Verification items for the finished model (mm, model axes). A direction names the side the tool comes from. Coordinates: 2 decimals unless noted, no trailing zeros. Order: outer loops, then holes, each group sorted by start corner. A loop starts at its lowest first (then second) coordinate and runs counter-clockwise, first axis right, second up. Notation, with made-up numbers: (53, 62) -> (69, 62) arc R18 ccw to (69, 92) -> close; hole circle Ø11 at (87, 42). An arc over 180 degrees is marked (long way). Write each question's results on one line, items separated by ' | '. Start each with the question number.
(1) Thickness scan on probe 1 along Y at (x, z) = (0, -8); probe 2 along Z at (x, y) = (2.5, -19.5); probe 3 along Y at (x, z) = (-33, -1.25). Record the ranges inside material, lowest first. Write a range as [from, to].
(2) Set-up check for faces 1 (the flat face through (0, 0, -14)), 2 (the cylindrical face through (0, 1, -9)), 3 (the flat face through (16, -25, -2)): record each of +Z, -Z, +X, -X, +Y, -Y from which the full face is reachable in a straight line by a thin tool's end or side.
(3) Cross-section at C-C on z = -1.5. Enter the section's corners in (x, y) (3 decimals).
(4) Cross-section at A-A on y = 0. Enter the section's corners in (x, z).
(5) Cross-section at D-D on z = -9. Enter the section's corners in (x, y), and give its area (3 significant figures).
(6) Go/stop test with flat-tipped pins: pin 1 (2 mm diameter, centred on y = -24, z = -1.5, fed in from +X); pin 2 (5 mm diameter, centred on y = -19, z = -1.5, fed in from -X); pin 3 (1 mm diameter, centred on x = 8.5, y = 10, fed in from -Z); pin 4 (1.8 mm diameter, centred on x = -30.094, y = 17.375, fed in from -Z). Record where each tip stops, or that it passes through.
(7) Draft check along X on faces 4 (the flat face through (-1, 1, 0)), 5 (the cylindrical face through (-31.593, -17.309, -1.972)), 6 (the cylindrical face through (-9, -40, -2)), 7 (the cylindrical face through (28.595, 17.441, -1.972)). Enter one of: +X half, -X half, draft (parallel to the pull), parting line (faces both ways), or undercut.
Autodesk Inventor part; units mm, degrees
ref_plane "Work Plane3" through (0, 0, 0) normal (0, 0, 1) x (1, 0, 0)
ref_plane "Work Plane6" through (0, 0, -4) normal (0, 0, -1) x (-1, 0, 0)
ref_plane "YZ Plane" through (0, 0, 0) normal (1, 0, 0) x (0, 1, 0)
sketch "Sketch1" plane through (0, 0, 0) normal (0, 0, 1) x (1, 0, 0)
  circle A0 centre (0, 0) radius 41
  circle A1 centre (0, 0) radius 17.705
  circle A2 centre (0, 0) radius 15
  circle A3 centre (0, 15) radius 0.75
  circle A4 centre (-10.6066, 10.6066) radius 0.75
  circle A5 centre (-15, 0) radius 0.75
  circle A6 centre (-10.6066, -10.6066) radius 0.75
  circle A7 centre (0, -15) radius 0.75
  circle A8 centre (10.6066, -10.6066) radius 0.75
  circle A9 centre (15, 0) radius 0.75
  circle A10 centre (10.6066, 10.6066) radius 0.75
  dimension "d4" = 30
  dimension "d0" = 82
  dimension "d3" = 35.41
  dimension "d5" = 1.5
  dimension "d6" = 360
sketch "Sketch2" plane through (0, 0, 0) normal (0, 0, 1) x (1, 0, 0)
  circle A0 centre (-30.094, -17.375) radius 1.5
  circle A1 centre (-30.094, 17.375) radius 1.5
  circle A2 centre (30.094, 17.375) radius 1.5
  circle A3 centre (30.094, -17.375) radius 1.5
  point P0 (0, 0)
  dimension "d7" = 3
  dimension "d8" = 3
  dimension "d9" = 3
  dimension "d10" = 3
  dimension "d11" = 17.375
  dimension "d12" = 30.094
  dimension "d13" = 30.094
  dimension "d14" = 17.375
  dimension "d15" = 17.375
  dimension "d16" = 30.094
  dimension "d17" = 17.375
  dimension "d18" = 30.094
extrude "Extrusion1" add sketch "Sketch1" against normal blind 4 contours A0 | A1 | A2 A9 | A2 A9 | A9 A2 A8 A7 A6 A5 A4 A3 A10 | A10 A2 | A2 A10 | A8 A2 | A2 A8 | A3 A2 | A2 A3 | A7 A2 | A2 A7 | A4 A2 | A2 A4 | A6 A2 | A2 A6 | A5 A2 | A2 A5
extrude "Extrusion2" cut sketch "Sketch2" against normal blind 4
ref_plane "Work Plane1" through (0, 0, -4) normal (0, 0, 1) x (1, 0, 0)
ref_plane "Work Plane2" through (0, 0, -4) normal (0, 0, 1) x (1, 0, 0)
ref_plane "Work Plane3" through (0, 0, 0) normal (0, 0, 1) x (1, 0, 0)
sketch "Sketch5" plane through (0, 0, 0) normal (0, 0, 1) x (1, 0, 0)
  line L0 (11, -30) -> (16, -30)
  line L1 (16, -30) -> (16, -20)
  line L2 (16, -20) -> (11, -20)
  line L3 (11, -20) -> (11, -30)
  point P0 (0, 0)
  point P1 (13.5, -20)
  point P2 (13.5, -30)
  point P3 (16, -25)
  dimension "d44" = 5
  dimension "d45" = 10
  dimension "d52" = 11
  dimension "d53" = 20
extrude "Extrusion5" cut sketch "Sketch5" against normal blind 4
fillet "Fillet1" radius 1.5 4 edges at (11, -20, -2) (11, -30, -2) (16, -20, -2) (16, -30, -2)
ref_plane "Work Plane6" through (0, 0, -4) normal (0, 0, -1) x (-1, 0, 0)
sketch "Sketch10" plane through (0, 0, -4) normal (0, 0, -1) x (-1, 0, 0)
  circle A0 centre (0, 0) radius 1
  dimension "d71" = 2
extrude "Extrusion10" add sketch "Sketch10" along normal blind 10
properties part number "lower-plate_3DPrint"
Results are:
1) probe 1: y = [-1, 1] | probe 2: z = [-4, 0] | probe 3: y = [-24.33, 24.33]
2) face 1: -Z, +X, -X, +Y, -Y | face 2: -Z | face 3: +Z, -Z
3) outline: circle Ø82 at (0, 0); hole circle Ø3 at (-30.094, -17.375); hole circle Ø3 at (-30.094, 17.375); hole (11, -28.5) arc R1.5 ccw to (12.5, -30) -> (14.5, -30) arc R1.5 ccw to (16, -28.5) -> (16, -21.5) arc R1.5 ccw to (14.5, -20) -> (12.5, -20) arc R1.5 ccw to (11, -21.5) -> close; hole circle Ø3 at (30.094, -17.375); hole circle Ø3 at (30.094, 17.375)
4) outline: (-41, -4) -> (-1, -4) -> (-1, -14) -> (1, -14) -> (1, -4) -> (41, -4) -> (41, 0) -> (-41, 0) -> close
5) outline: circle Ø2 at (0, 0) | area: 3.14 mm2
6) pin 1: stops at x = 33.94 | pin 2: stops at x = -37.53 | pin 3: stops at z = -4 | pin 4: passes through
7) face 4: draft | face 5: undercut | face 6: parting line | face 7: undercut
